```python
from build123d import *

# Parameters (mm, degrees)
SKETCH1_W           = 20
SKETCH1_H           = 41.1
SKETCH1_W_2         = 20.2
SKETCH1_H_2         = 41.3
SKETCH1_W_3         = 20.4
SKETCH1_H_3         = 41.5
BOSS_EXTRUDE1_DEPTH = 5


with BuildPart() as part:
    # Sketch1 → Boss-Extrude1 (new body)
    with BuildSketch(Plane(origin=(0, 0, 0), x_dir=(1, 0, 0), z_dir=(0, 1, 0))):
        with BuildLine():
            Line((-2.5, -25.15), (-2.5, -24.15))
            ThreePointArc((-2.5, -24.15), (-2.353553391, -23.796446609), (-2, -23.65))
            Line((-2, -23.65), (2, -23.65))
            ThreePointArc((2, -23.65), (2.353553391, -23.796446609), (2.5, -24.15))
            Line((2.5, -24.15), (2.5, -25.15))
            ThreePointArc((2.5, -25.15), (2.646446609, -25.503553391), (3, -25.65))
            Line((3, -25.65), (63.2, -25.65))
            ThreePointArc((63.2, -25.65), (64.614213562, -25.064213562), (65.2, -23.65))
            Line((65.2, -23.65), (65.2, 23.65))
            ThreePointArc((65.2, 23.65), (64.614213562, 25.064213562), (63.2, 25.65))
            Line((63.2, 25.65), (-13, 25.65))
            ThreePointArc((-13, 25.65), (-14.414213562, 25.064213562), (-15, 23.65))
            Line((-15, 23.65), (-15, -23.65))
            ThreePointArc((-15, -23.65), (-14.414213562, -25.064213562), (-13, -25.65))
            Line((-13, -25.65), (-3, -25.65))
            ThreePointArc((-3, -25.65), (-2.646446609, -25.503553391), (-2.5, -25.15))
        make_face()
        Rectangle(SKETCH1_W, SKETCH1_H, mode=Mode.SUBTRACT)
        with Locations((25.1, 0)):
            Rectangle(SKETCH1_W_2, SKETCH1_H_2, mode=Mode.SUBTRACT)
        with Locations((50.4, 0)):
            Rectangle(SKETCH1_W_3, SKETCH1_H_3, mode=Mode.SUBTRACT)
    extrude(amount=BOSS_EXTRUDE1_DEPTH)


solid = part.part
```
CAD build for the part. Positions are in the model's coordinates, mm. A direction names the side the tool comes from. Give positions to 0.01 mm unless a question says otherwise; leave off trailing zeros. Order: outer loops, then holes, each group sorted by start corner. A loop starts at its lowest first (then second) coordinate and runs counter-clockwise, first axis right, second up.
(1) Flat gauge pins, fed straight in: pin 1 (3 mm diameter, centred on x = 0.5, y = 2, fed in from +Z); pin 2 (0.8 mm diameter, centred on y = 3.5, z = 24.5, fed in from -X); pin 3 (1.1 mm diameter, centred on y = 2.5, z = 25, fed in from +X). Where does each tip first touch, or does it go through?
(2) Saw through at C-C, the plane y = 3.4. Give the cut face in (x, z), then the cut area to 3 significant figures.
(3) Tool access for faces 4 (the flat face through (15, 2, 0)), 5 (the flat face through (26, 2, -25.65)), 6 (the flat face through (0, 2, 23.65)): list every direction of +Z, -Z, +X, -X, +Y, -Y with a clear straight run to the whole face (end or side of a thin tool).
(4) Drill centre lines: L1, parallel to X at y = 0.35, z = -4.5; L2, parallel to Z at x = 6, y = 4.4; L3, parallel to Z at x = 43.5, y = 0.75. Where is each one in solid material? Low to high.
(5) Mould opens along Z. For faces 1 (the cylindrical face through (-14.4, 2.46, -25.08)), 2 (the flat face through (35.2, 2, 0)), 3 (the cylindrical face through (64.6, 2.46, 25.08)) say: released by +Z, released by -Z, zero draft, split by the parting line, or undercut.
(6) Saw through at A-A, the plane x = 30.5. Give the cut face in (y, z).
(7) Saw through at D-D, the plane x = 58. Give the cut face in (y, z), then the cut area to 3 significant figures.
(8) Saw through at B-B, the plane z = 16.5. Give the cut face in (x, y).
Results found:
1. pin 1: stops at z = 23.65
1. pin 2: stops at x = -14.95
1. pin 3: stops at x = 65.03
2. outline: (-15, -23.65) arc R2 ccw to (-13, -25.65) - (63.2, -25.65) arc R2 ccw to (65.2, -23.65) - (65.2, 23.65) arc R2 ccw to (63.2, 25.65) - (3, 25.65) arc R0.5 ccw to (2.5, 25.15) - (2.5, 24.15) arc R0.5 cw to (2, 23.65) - (-2, 23.65) arc R0.5 cw to (-2.5, 24.15) - (-2.5, 25.15) arc R0.5 ccw to (-3, 25.65) - (-13, 25.65) arc R2 ccw to (-15, 23.65) - close; hole (-10, -20.55) - (10, -20.55) - (10, 20.55) - (-10, 20.55) - close; hole (15, -20.65) - (35.2, -20.65) - (35.2, 20.65) - (15, 20.65) - close; hole (40.2, -20.75) - (60.6, -20.75) - (60.6, 20.75) - (40.2, 20.75) - close
2. area: 1,600 mm2
3. face 4: +Y, -Y
3. face 5: -Z, +X, -X, +Y, -Y
3. face 6: +Z, +Y, -Y
4. L1: x = -15 to -10, 10 to 15, 35.2 to 40.2, 60.6 to 65.2
4. L2: z = -25.65 to -20.55, 20.55 to 25.65
4. L3: z = -25.65 to -20.75, 20.75 to 25.65
5. face 1: released by -Z
5. face 2: undercut
5. face 3: released by +Z
6. outline: (0, -25.65) - (5, -25.65) - (5, -20.65) - (0, -20.65) - close; (0, 20.65) - (5, 20.65) - (5, 25.65) - (0, 25.65) - close
7. outline: (0, -25.65) - (5, -25.65) - (5, -20.75) - (0, -20.75) - close; (0, 20.75) - (5, 20.75) - (5, 25.65) - (0, 25.65) - close
7. area: 49.0 mm2
8. outline: (-15, 0) - (-10, 0) - (-10, 5) - (-15, 5) - close; (10, 0) - (15, 0) - (15, 5) - (10, 5) - close; (35.2, 0) - (40.2, 0) - (40.2, 5) - (35.2, 5) - close; (60.6, 0) - (65.2, 0) - (65.2, 5) - (60.6, 5) - close
